Model file for the job. Use its own axes, mm. Face numbers are marked on the shaded views. A direction names the side the tool comes from. Round coordinates to 2 decimals unless told otherwise and drop trailing zeros. Order: outer loops, then holes, each group sorted by start corner. A loop starts at its lowest first (then second) coordinate and runs counter-clockwise, first axis right, second up. Notation, with made-up numbers: M -31.75,88.5 L -13.75,88.5 A18 ccw -13.75,99.5 Z; hole C 19.5,27 d9. An arc over 180 degrees is marked long. Return JSON: item names as keys, results as strings. Group by question number.
Item 1: Which spindle directions (+Z, -Z, +X, -X, +Y, -Y) get a long thin tool onto all of the face, cutting with end or side? Do the marked faces 4, 5 and 6. Say none if no direction does.
Item 2: Slice it at B-B on z = 54.5. Write the cut outline in (x, y).
Item 3: Slice it at C-C on z = 149.5. Write the cut outline in (x, y).
Item 4: Pin check, flat tips, straight feed: pin 1 Ø8 at (x, y) = (97, -26.5) entering from -Z; pin 2 Ø4 at (x, y) = (175.5, -79) entering from +Z; pin 3 Ø1.5 at (y, z) = (-63.5, 169.5) entering from -X. Stop position of each tip, or through.
Item 5: Probe line 1 along Z through (x, y) = (145, -35.5); line 2 along Z through (x, y) = (194, 28.5); line 3 along Y through (x, z) = (51.5, -27). List the from-to ranges inside material, lowest first.
Item 6: Slice it at A-A on x = 101.6. Write the cut outline in (y, z).
Item 7: Pull direction Z, two halves, no side cores. Call the marked faces 1, 2 and 3: pulls with the +Z half, pulls with the -Z half, needs draft (parallel to the pull), parting line crosses it, or undercut.
from build123d import *

# Parameters (mm, degrees)
F1_DEPTH = 203.2
F2_R     = 40.64
F3_DEPTH = 635
F4_R     = 86.36
F5_DEPTH = 101.6
F6_SIZE2 = 7.62
F6_SIZE  = 7.62
F7_SIZE2 = 5.08
F7_SIZE  = 5.08


with BuildPart() as f1:
    # F0 (on Right) → F1 (new body)
    with BuildSketch(Plane.YZ):
        Polygon((-101.3922498733, -72.2344086301), (-50.5922498733, -72.2344086301), (-50.5922498733, 59.8455913699), (101.8077501267, 59.8455913699), (101.8077501267, 110.6455913699), (-101.3922498733, 110.6455913699), align=None)
    extrude(amount=F1_DEPTH)

    # F2 (on face) → F3 (cut)
    with BuildSketch(Plane.XZ.offset(101.3922498733)):
        with Locations((101.6, -6.1944086301)):
            Circle(F2_R)
    extrude(amount=-F3_DEPTH, mode=Mode.SUBTRACT)

    # F4 (on face) → F5 (join)
    with BuildSketch(Plane.XY.offset(110.6455913699)):
        with Locations((101.6, 0.2077501267)):
            Circle(F4_R)
    extrude(amount=F5_DEPTH)

    # F6
    f6_edges = [f1.edges().sort_by_distance(p)[0] for p in [
        (15.24, 0.20775, 212.245591),
    ]]
    chamfer(f6_edges, length=F6_SIZE, length2=F6_SIZE2)

    # F7
    f7_edges = [f1.edges().sort_by_distance(p)[0] for p in [
        (60.96, -101.39225, -6.194409),
        (60.96, -50.59225, -6.194409),
    ]]
    chamfer(f7_edges, length=F7_SIZE, length2=F7_SIZE2)


solid = f1.part
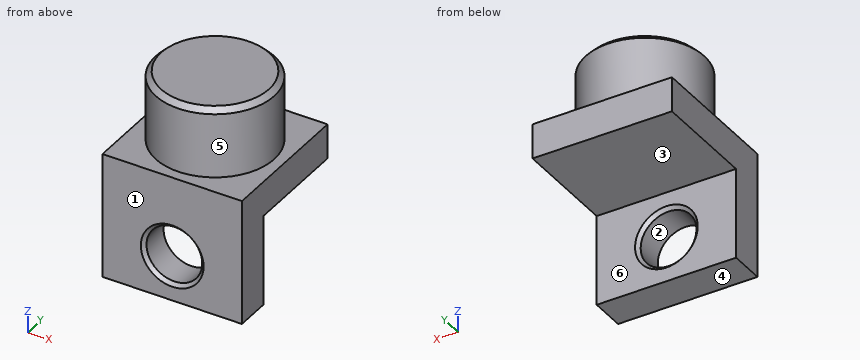
Output values:
{
 "1": {"face 4": "-Z, +X, -X, +Y, -Y", "face 5": "+Z", "face 6": "-Z, +X, -X, +Y"},
 "2": {"outline": "M 0,-101.39 L 203.2,-101.39 L 203.2,-50.59 L 0,-50.59 Z"},
 "3": {"outline": "C 101.6,0.21 d172.72"},
 "4": {"pin 1": "z = 59.85", "pin 2": "z = 110.65", "pin 3": "x = 42.49"},
 "5": {"line 1": "59.85 to 212.25", "line 2": "59.85 to 110.65", "line 3": "-101.39 to -50.59"},
 "6": {"outline": "M -101.39,-72.23 L -50.59,-72.23 L -50.59,-51.91 L -55.67,-46.83 L -96.31,-46.83 L -101.39,-51.91 Z; M -101.39,39.53 L -96.31,34.45 L -55.67,34.45 L -50.59,39.53 L -50.59,59.85 L 101.81,59.85 L 101.81,110.65 L 86.57,110.65 L 86.57,204.63 L 78.95,212.25 L -78.53,212.25 L -86.15,204.63 L -86.15,110.65 L -101.39,110.65 Z"},
 "7": {"face 1": "needs draft", "face 2": "undercut", "face 3": "pulls with the -Z half"}
}
